from build123d import *

# Parameters (mm, degrees)
BOSS_EXTRUDE1_DEPTH = 45
SKETCH2_W           = 20.5
SKETCH2_H           = 2
BOSS_EXTRUDE2_DEPTH = 18.5
SKETCH3_W           = 20.5
SKETCH3_H           = 3.5
CUT_EXTRUDE1_DEPTH  = 20
SKETCH4_W           = 20.5
SKETCH4_H           = 3
BOSS_EXTRUDE3_DEPTH = 43.25


with BuildPart() as part:
    # Sketch1 → Boss-Extrude1 (new body)
    with BuildSketch(Plane(origin=(0, 0, 0), x_dir=(1, 0, 0), z_dir=(0, 1, 0))):
        Polygon((0, 0), (26.5, 0), (34.916811667, 23.125), (26.5, 46.25), (23.5, 46.25), (23.5, 3), (3, 3), (3, 46.25), (0, 46.25), (-8.416811667, 23.125), align=None)
    extrude(amount=BOSS_EXTRUDE1_DEPTH)

    # Sketch2 → Boss-Extrude2 (add)
    with BuildSketch(Plane(origin=(0, 0, -3), x_dir=(-1, 0, 0), z_dir=(0, 0, -1))):
        with Locations((-13.25, 44)):
            Rectangle(SKETCH2_W, SKETCH2_H)
    extrude(amount=BOSS_EXTRUDE2_DEPTH)

    # Sketch3 → Cut-Extrude1 (cut)
    with BuildSketch(Plane(origin=(0, 0, -3), x_dir=(-1, 0, 0), z_dir=(0, 0, -1))):
        with Locations((-13.25, 32)):
            Rectangle(SKETCH3_W, SKETCH3_H)
    extrude(amount=-CUT_EXTRUDE1_DEPTH, mode=Mode.SUBTRACT)

    # Sketch4 → Boss-Extrude3 (add)
    with BuildSketch(Plane(origin=(0, 0, -3), x_dir=(-1, 0, 0), z_dir=(0, 0, -1))):
        with Locations((-13.25, 1.5)):
            Rectangle(SKETCH4_W, SKETCH4_H)
    extrude(amount=BOSS_EXTRUDE3_DEPTH)


solid = part.part
Can you work these out from the model? Positions are in its coordinate system, mm. A direction names the side the tool comes from. Coordinates: 2 decimals unless noted, no trailing zeros. Write each loop counter-clockwise with the first axis right and the second up, starting at its lowest first coordinate (ties: lowest second). Pieces come first, ordered by that corner, then holes.
Q1. Imagine slicing it at C-C, the plane y = 16. List the corners of the cut face in (x, z) for me (3 decimals).
Results found:
outline: (-8.417, -23.125) - (0, -46.25) - (3, -46.25) - (3, -3) - (23.5, -3) - (23.5, -46.25) - (26.5, -46.25) - (34.917, -23.125) - (26.5, 0) - (0, 0) - close
Q2. For P1, Ø1.5, axis at x = 12, z = -2, coming from the -Y side; P2, Ø1.6, axis at x = 12, y = 44, coming from the -Z side; P3, Ø4.5, axis at x = 16.5, y = 38, coming from the -Z side; P4, Ø6, axis at y = 11.5, z = -23, coming from the +X side, each with a flat end and sliding along its axis, tell me the tip position at first contact or that it passes through.
Results found:
P1: stops at y = 0
P2: stops at z = -21.5
P3: stops at z = -3
P4: stops at x = 34.92
Q3. Imagine slicing it at D-D, the plane z = -32.5. List the corners of the cut face in (x, y) for me.
Results found:
outline: (-5, 0) - (31.5, 0) - (31.5, 45) - (23.5, 45) - (23.5, 3) - (3, 3) - (3, 45) - (-5, 45) - close
Q4. Imagine slicing it at B-B, the plane z = -18. List the corners of the cut face in (x, y) for me, plus the area to 3 significant figures.
Results found:
outline: (-6.55, 0) - (33.05, 0) - (33.05, 45) - (-6.55, 45) - close; hole (3, 3) - (23.5, 3) - (23.5, 43) - (3, 43) - close
area: 962 mm2
Q5. If we mould it in two halves opening along X, with no side actions, what happens to faces 4 (the face through (30.65, 22.18, -11.4)), 5 (the face through (13, 45, -18)), 6 (the face through (13, 16, -3))? For each: +X half, -X half, draft (parallel to the pull), parting line (faces both ways), or undercut.
Results found:
face 4: +X half
face 5: draft
face 6: undercut
Q6. Imagine slicing it at A-A, the plane x = 11.5. List the corners of the cut face in (y, z) for me.
Results found:
outline: (0, -46.25) - (3, -46.25) - (3, -3) - (30.25, -3) - (30.25, 0) - (0, 0) - close; (33.75, -3) - (43, -3) - (43, -21.5) - (45, -21.5) - (45, 0) - (33.75, 0) - close
Q7. Which directions (+Z, -Z, +X, -X, +Y, -Y) give clear straight access to the entire face, cutting with the end or side of a thin tool? Please do faces 1 (the face through (13, 44, -21.5)), 2 (the face through (13, 30.25, -2)), 3 (the face through (13, 43, -12)).
Results found:
face 1: -Z, +Y
face 2: +Z, -Z
face 3: -Z
Q8. Please list where these lines run through material, in increasing order: L1, parallel to Y at x = 22.5, z = -4; L2, parallel to X at y = 41, z = -25; L3, parallel to Z at x = 12.5, y = 13.
Results found:
L1: y = 0 to 3, 43 to 45
L2: x = -7.73 to 3, 23.5 to 34.23
L3: z = -3 to 0
